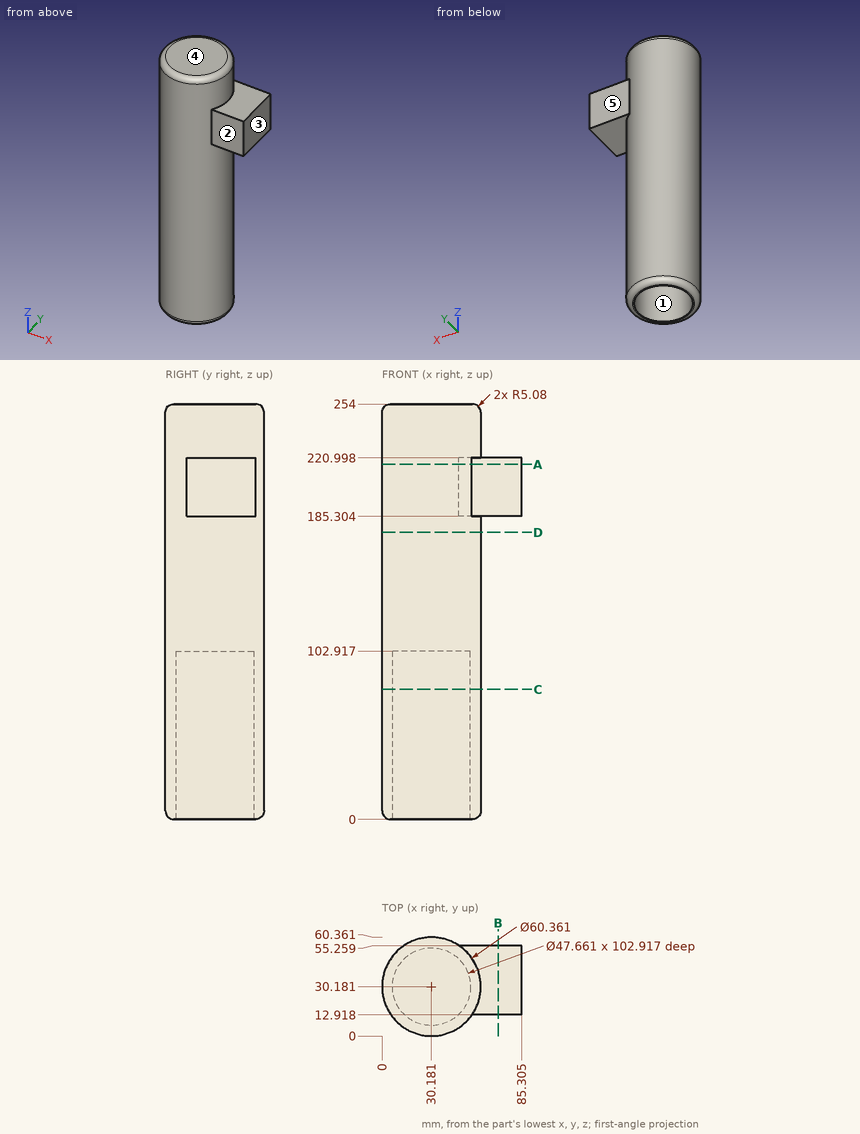
The drawing under review shows one solid part. Ordinate dimensions are in mm from its lowest x, y, z. A direction names the side the tool comes from. Round coordinates to 2 decimals unless told otherwise and drop trailing zeros. Loops run counter-clockwise (first coordinate to the right, second up) from the corner with the lowest first, then second, coordinate; pieces in that order, holes last. Notation, with made-up numbers: (21.25, 9) - (39.25, 9) arc R10 cw to (39.25, 17) - close; hole circle Ø3 at (-13, 32). An arc over 180 degrees is marked (long way). Put each result on its own line as item: value. Start each with the question number.
1. Insertion check: P1, Ø12, axis at x = 75.5, y = 7, coming from the -Z side; P2, Ø24.5, axis at x = 67.5, z = 209.5, coming from the -Y side; P3, Ø11.5, axis at x = 73.5, y = 29, coming from the +Z side. Each pin has a flat end and moves straight along its axis. Give the tip position at first contact, or say it passes through.
2. Consider section C-C on z = 79.5. State the section outline as (x, y) points.
3. For probe 1 along Z at (x, y) = (61, 22); probe 2 along Z at (x, y) = (37, 12); probe 3 along X at (y, z) = (17, 32) (1 decimal), list the stretches that pass through material, from the lowest coordinate up. Write a range as [from, to].
4. Consider section B-B on x = 71. State the section outline as (y, z) points.
5. For the marked faces 4 and 5, list the 3-axis set-ups (+Z, -Z, +X, -X, +Y, -Y) from which the entire face can be reached by the end or side of a thin tool; tool diameter is ignored.
6. Mouldability with a two-part tool opening along Y and no side actions: class the marked faces 1, 2 and 3 as +Y half, -Y half, draft (parallel to the pull), parting line (faces both ways), or undercut.
7. Consider section D-D on z = 175.5. State the section outline as (x, y) points, plus the area to 3 significant figures.
8. Consider section A-A on z = 217. State the section outline as (x, y) points (1 decimal).
Result sheet:
1. P1: z = 185.3
1. P2: y = 12.92
1. P3: z = 221
2. outline: circle Ø60.36 at (30.18, 30.18); hole circle Ø47.66 at (30.18, 30.18)
3. probe 1: [185.3, 221]
3. probe 2: [102.92, 254]
3. probe 3: [3, 10.3], [50, 57.3]
4. outline: (12.92, 185.3) - (55.26, 185.3) - (55.26, 221) - (12.92, 221) - close
5. face 4: +Z, +X, -X, +Y, -Y
5. face 5: +Z, -Z, +X, +Y
6. face 1: undercut
6. face 2: -Y half
6. face 3: draft
7. outline: circle Ø60.36 at (30.18, 30.18)
7. area: 2,860 mm^2
8. outline: (47, 55.3) arc R30.2 ccw (long way) to (54.9, 12.9) - (85.3, 12.9) - (85.3, 55.3) - close
